```python
from build123d import *

# Parameters (mm, degrees)
F1_DEPTH = 10
F2_DEPTH = 35
F0_W     = 10
F0_H     = 15
F3_DEPTH = 35
F0_W_2   = 30
F0_H_2   = 5
F4_DEPTH = 35


with BuildPart() as f1:
    # F0 (on Front) → F1 (new body)
    with BuildSketch(Plane.XZ):
        Polygon((-22.5, -20), (32.5, -20), (32.5, 0), (-7.5, 20), (-32.5, 20), (-32.5, 15), (-22.5, 15), (-22.5, 0), (-22.5, -8.847731), (7.5, -8.847731), (7.5, -13.847731), (-22.5, -13.847731), align=None)
    extrude(amount=F1_DEPTH)

    # F0 (on Front) → F2 (join)
    with BuildSketch(Plane.XZ):
        Polygon((-32.5, -20), (-22.5, -20), (-22.5, -13.847731), (-22.5, -8.847731), (-22.5, 0), (-32.5, 0), align=None)
    extrude(amount=F2_DEPTH)

    # F0 (on Front) → F3 (join)
    with BuildSketch(Plane.XZ):
        with Locations((-27.5, 7.5)):
            Rectangle(F0_W, F0_H)
    extrude(amount=F3_DEPTH)

    # F0 (on Front) → F4 (join)
    with BuildSketch(Plane.XZ):
        with Locations((-7.5, -11.347731)):
            Rectangle(F0_W_2, F0_H_2)
    extrude(amount=F4_DEPTH)


solid = f1.part
```
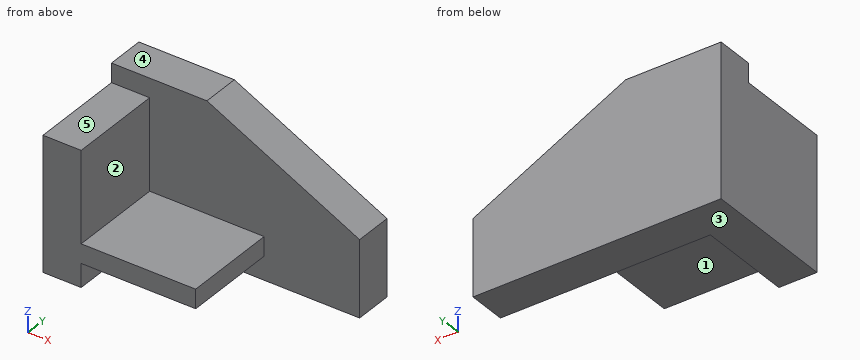
Model file for the job. Use its own axes, mm. Face numbers are marked on the shaded views. A direction names the side the tool comes from. Give positions to 0.01 mm unless a question says otherwise; leave off trailing zeros. Order: outer loops, then holes, each group sorted by start corner. A loop starts at its lowest first (then second) coordinate and runs counter-clockwise, first axis right, second up.
1) Saw through at C-C, the plane x = -15.5. Write the cut outline in (y, z).
2) 3-axis set-ups, long thin cutter, end or side, ignore diameter. For the marked faces 1, 2, 3, 4 and 5: which of +Z, -Z, +X, -X, +Y, -Y reach the whole face in a straight line?
3) Saw through at A-A, the plane y = -15. Write the cut outline in (x, z).
4) Saw through at B-B, the plane z = 8.5. Write the cut outline in (x, y), then the cut area to 3 significant figures.
5) Saw through at D-D, the plane y = -9. Write the cut outline in (x, z), then the cut area to 3 significant figures.
6) Pin check, flat tips, straight feed: pin 1 (2.5 mm diameter, centred on y = -18, z = -10, fed in from +X); pin 2 (4 mm diameter, centred on x = 6, y = -22, fed in from -Z); pin 3 (12 mm diameter, centred on x = -12.5, z = 5, fed in from -Y). Stop position of each tip, or through.
7) Wall check: probe 1 along Y at (x, z) = (-5.5, 3); probe 2 along Z at (x, y) = (-1, -27); probe 3 along X at (y, z) = (-19, 9.5). Give the ranges that are in metal, low to high.
Computed:
1. outline: (-35, -13.85) - (-10, -13.85) - (-10, -20) - (0, -20) - (0, 20) - (-10, 20) - (-10, -8.85) - (-35, -8.85) - close
2. face 1: -Z, +X, -Y
2. face 2: +Z, +X, -Y
2. face 3: -Z, +X, -X, +Y, -Y
2. face 4: +Z, +X, -X, +Y, -Y
2. face 5: +Z, +X, -X, -Y
3. outline: (-32.5, -20) - (-22.5, -20) - (-22.5, -13.85) - (7.5, -13.85) - (7.5, -8.85) - (-22.5, -8.85) - (-22.5, 15) - (-32.5, 15) - close
4. outline: (-32.5, -35) - (-22.5, -35) - (-22.5, -10) - (15.5, -10) - (15.5, 0) - (-32.5, 0) - close
4. area: 730 mm2
5. outline: (-32.5, -20) - (32.5, -20) - (32.5, 0) - (-7.5, 20) - (-32.5, 20) - close
5. area: 2,200 mm2
6. pin 1: stops at x = 7.5
6. pin 2: stops at z = -13.85
6. pin 3: stops at y = -10
7. probe 1: y = -10 to 0
7. probe 2: z = -13.85 to -8.85
7. probe 3: x = -32.5 to -22.5
